For this review, take the finished solid that the model builds, in its own axes (mm). Coordinates: 2 decimals unless noted, no trailing zeros. Order: outer loops, then holes, each group sorted by start corner. A loop starts at its lowest first (then second) coordinate and runs counter-clockwise, first axis right, second up. Notation, with made-up numbers: (25.25, 71.5) -> (32.25, 71.5) arc R20 ccw to (32.25, 98.5) -> close; hole circle Ø5 at (75.25, 85). An arc over 180 degrees is marked (long way). Answer as a JSON object with one key per item and string values. Group by question number.
1) Draft analysis for pull direction Y (two halves, no side actions). For faces 1 (the cylindrical face through (-26.75, 257.82, 4.93)), 2 (the cylindrical face through (-18.445, 22.259, 4.93)), 3 (the flat face through (-42, 106, 5)), state which applies: +Y half, -Y half, draft (parallel to the pull), parting line (faces both ways), or undercut.
2) Add section C-C, the plane x = 24. Write out the cut boundary in (y, z), then the cut area to 3 significant figures.
3) Add section A-A, the plane z = 1.5. Write out the cut boundary in (x, y), then the cut area to 3 significant figures.
4) Add section B-B, the plane y = 18. Write out the cut boundary in (x, z).
5) Wall thickness on L1, parallel to X at y = 20, z = 8; L2, parallel to Y at x = -24, z = 4; L3, parallel to Y at x = 19, z = 6.5: over which ranges is each line inside the solid? List them lowest first.
6) For pin 1 (2 mm diameter, centred on y = 232.5, z = 1.5, fed in from -X); pin 2 (11 mm diameter, centred on x = -24, y = 18, fed in from -Z), all flat-tipped, find the tip position at first contact; note any pin that passes through.
from build123d import *

# Parameters (mm, degrees)
SKETCH1_R           = 7
BOSS_EXTRUDE1_DEPTH = 10


with BuildPart() as part:
    # Sketch1 → Boss-Extrude1 (new body)
    with BuildSketch(Plane.XY):
        with BuildLine():
            Line((-20.517714388, 260), (20.517714388, 260))
            ThreePointArc((20.517714388, 260), (26.67774114, 257.877440601), (30.222763355, 252.410814084))
            Line((30.222763355, 252.410814084), (42, 205))
            Line((42, 205), (42, 10))
            ThreePointArc((42, 10), (39.071067812, 2.928932188), (32, 0))
            Line((32, 0), (-32, 0))
            ThreePointArc((-32, 0), (-39.071067812, 2.928932188), (-42, 10))
            Line((-42, 10), (-42, 205))
            Line((-42, 205), (-30.222763355, 252.410814084))
            ThreePointArc((-30.222763355, 252.410814084), (-26.67774114, 257.877440601), (-20.517714388, 260))
        make_face()
        with Locations((24, 18)):
            Circle(SKETCH1_R, mode=Mode.SUBTRACT)
        with Locations(Location((-24, 18, 0), (0, 0, 180))):
            Circle(SKETCH1_R, mode=Mode.SUBTRACT)
    extrude(amount=BOSS_EXTRUDE1_DEPTH)


solid = part.part
Output values:
{
 "1": {"face 1": "+Y half", "face 2": "undercut", "face 3": "draft"},
 "2": {"outline": "(0, 0) -> (11, 0) -> (11, 10) -> (0, 10) -> close; (25, 0) -> (259.37, 0) -> (259.37, 10) -> (25, 10) -> close", "area": "2,450 mm²"},
 "3": {"outline": "(-42, 10) arc R10 ccw to (-32, 0) -> (32, 0) arc R10 ccw to (42, 10) -> (42, 205) -> (30.22, 252.41) arc R10 ccw to (20.52, 260) -> (-20.52, 260) arc R10 ccw to (-30.22, 252.41) -> (-42, 205) -> close; hole circle Ø14 at (-24, 18); hole circle Ø14 at (24, 18)", "area": "20,700 mm²"},
 "4": {"outline": "(-42, 0) -> (-31, 0) -> (-31, 10) -> (-42, 10) -> close; (-17, 0) -> (17, 0) -> (17, 10) -> (-17, 10) -> close; (31, 0) -> (42, 0) -> (42, 10) -> (31, 10) -> close"},
 "5": {"L1": "x = -42 to -30.71, -17.29 to 17.29, 30.71 to 42", "L2": "y = 0 to 11, 25 to 259.37", "L3": "y = 0 to 13.1, 22.9 to 260"},
 "6": {"pin 1": "stops at x = -35.42", "pin 2": "passes through"}
}
